Model file for the job. Use its own axes, mm. Face numbers are marked on the shaded views. A direction names the side the tool comes from. Round coordinates to 2 decimals unless told otherwise and drop trailing zeros. Order: outer loops, then holes, each group sorted by start corner. A loop starts at its lowest first (then second) coordinate and runs counter-clockwise, first axis right, second up. Notation, with made-up numbers: M 82,79.5 L 119,79.5 A28 ccw 119,104.5 Z; hole C 38.5,78 d7. An arc over 180 degrees is marked long. Return JSON: item names as keys, results as strings. Group by question number.
Item 1: Slice it at C-C on z = 10. Write the cut outline in (x, y), then the cut area to 3 significant figures.
Item 2: Slice it at D-D on x = 19. Write the cut outline in (y, z).
Item 3: Slice it at B-B on x = 40. Write the cut outline in (y, z), then the cut area to 3 significant figures.
Item 4: Pin check, flat tips, straight feed: pin 1 Ø2 at (x, z) = (10, 5) entering from +Y; pin 2 Ø8 at (x, z) = (0, 0) entering from +Y; pin 3 Ø1.8 at (x, z) = (1, 1) entering from +Y. Stop position of each tip, or through.
Item 5: Which spindle directions (+Z, -Z, +X, -X, +Y, -Y) get a long thin tool onto all of the face, cutting with end or side? Do the marked faces 1, 2, 3 and 4. Say none if no direction does.
Item 6: Slice it at A-A on y = 2.5. Write the cut outline in (x, z), then the cut area to 3 significant figures.
Item 7: Probe line 1 along X through (y, z) = (4.7, 0); line 2 along X through (y, z) = (4.45, 0); line 3 along Z through (x, y) = (40, 1.65). List the from-to ranges inside material, lowest first.
Item 8: Pull direction X, two halves, no side cores. Call the marked faces 5, 6, 7 and 8: pulls with the +X half, pulls with the -X half, needs draft (parallel to the pull), parting line crosses it, or undercut.
from build123d import *

# Parameters (mm, degrees)
EXTRUDE_1_DEPTH     = 4
SKETCH_2_R          = 4.5
SKETCH_2_R_2        = 3
EXTRUDE_2_DEPTH     = 2.5
EXTRUDE_3_DEPTH     = 25
SKETCH_4_W          = 7
SKETCH_4_H          = 5
CUT_EXTRUDE_1_DEPTH = 57.621550668
SKETCH_5_W          = 7
SKETCH_5_H          = 5
CUT_EXTRUDE_2_DEPTH = 52.780787943
EXTRUDE_4_DEPTH     = 2
SKETCH_7_R          = 3
SKETCH_7_R_2        = 1.5
EXTRUDE_5_DEPTH     = 1


with BuildPart() as part:
    # 草图1 → 凸台-拉伸1 (new body)
    with BuildSketch(Plane(origin=(0, 0, 0), x_dir=(1, 0, 0), z_dir=(0, 1, 0))):
        with BuildLine():
            ThreePointArc((12.5, 0), (8.838834765, 8.838834765), (0, 12.5))
            ThreePointArc((0, 12.5), (-8.838834765, 8.838834765), (-12.5, 0))
            Line((-12.5, 0), (-1.5, 0))
            ThreePointArc((-1.5, 0), (0, 1.5), (1.5, 0))
            Line((1.5, 0), (12.5, 0))
        make_face()
        with BuildLine():
            ThreePointArc((0, -12.5), (8.838834765, -8.838834765), (12.5, 0))
            Line((12.5, 0), (1.5, 0))
            ThreePointArc((1.5, 0), (0, -1.5), (-1.5, 0))
            Line((-1.5, 0), (-12.5, 0))
            ThreePointArc((-12.5, 0), (-8.838834765, -8.838834765), (0, -12.5))
        make_face()
        with BuildLine():
            Line((50, 12.5), (0, 12.5))
            ThreePointArc((0, 12.5), (8.838834765, 8.838834765), (12.5, 0))
            Line((12.5, 0), (38.5, 0))
            ThreePointArc((38.5, 0), (40, 1.5), (41.5, 0))
            Line((41.5, 0), (50, 0))
            Line((50, 0), (50, 12.5))
        make_face()
        with BuildLine():
            Line((38.5, 0), (12.5, 0))
            ThreePointArc((12.5, 0), (8.838834765, -8.838834765), (0, -12.5))
            Line((0, -12.5), (50, -12.5))
            Line((50, -12.5), (50, 0))
            Line((50, 0), (41.5, 0))
            ThreePointArc((41.5, 0), (40, -1.5), (38.5, 0))
        make_face()
    extrude(amount=EXTRUDE_1_DEPTH)

    # 草图2 → 凸台-拉伸2 (add)
    with BuildSketch(Plane(origin=(0, 4, 0), x_dir=(1, 0, 0), z_dir=(0, 1, 0))):
        with Locations(Location((0, 0, 0), (0, 0, 270))):
            Circle(SKETCH_2_R)
        with Locations(Location((0, 0, 0), (0, 0, 270))):
            Circle(SKETCH_2_R_2, mode=Mode.SUBTRACT)
    extrude(amount=EXTRUDE_2_DEPTH)

    # 草图3 → 凸台-拉伸3 (add)
    with BuildSketch(Plane.XY.offset(12.5)):
        Polygon((33, 9), (47, 9), (50, 4), (30, 4), align=None)
    extrude(amount=-EXTRUDE_3_DEPTH)

    # 草图4 → 切除-拉伸1 (cut, through all)
    with BuildSketch(Plane.XY.offset(12.5)):
        with Locations((40, 6.5)):
            Rectangle(SKETCH_4_W, SKETCH_4_H)
    extrude(amount=-CUT_EXTRUDE_1_DEPTH, mode=Mode.SUBTRACT)

    # 草图5 → 切除-拉伸2 (cut, through all)
    with BuildSketch(Plane(origin=(0, 4, 0), x_dir=(1, 0, 0), z_dir=(0, 1, 0))):
        with Locations((40, -10)):
            Rectangle(SKETCH_5_W, SKETCH_5_H)
        with Locations((40, 10)):
            Rectangle(SKETCH_5_W, SKETCH_5_H)
    extrude(amount=-CUT_EXTRUDE_2_DEPTH, mode=Mode.SUBTRACT)

    # 草图6 → 凸台-拉伸4 (add, symmetric)
    with BuildSketch(Plane.XY):
        Polygon((30, 4), (33, 9), (4.5, 6.5), (3.215772895, 6.5), (3.215772895, 4), align=None)
    extrude(amount=EXTRUDE_4_DEPTH, both=True)

    # 草图7 → 凸台-拉伸5 (add)
    with BuildSketch(Plane(origin=(0, 4, 0), x_dir=(1, 0, 0), z_dir=(0, 1, 0))):
        with Locations(Location((0, 0, 0), (0, 0, 270))):
            Circle(SKETCH_7_R)
        with Locations(Location((0, 0, 0), (0, 0, 270))):
            Circle(SKETCH_7_R_2, mode=Mode.SUBTRACT)
    extrude(amount=EXTRUDE_5_DEPTH)


solid = part.part
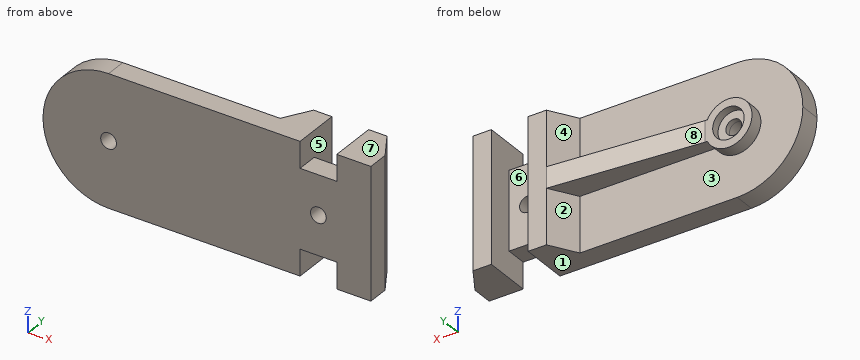
Output values:
{
 "1": {"outline": "M -7.5,0 L 36.5,0 L 36.5,9 L 33,9 L 30,4 L -7.5,4 Z; M 43.5,0 L 50,0 L 50,4 L 47,9 L 43.5,9 Z", "area": "252 mm²"},
 "2": {"outline": "M 0,-12.5 L 4,-12.5 L 4,-2 L 7.77,-2 L 7.77,2 L 4,2 L 4,12.5 L 0,12.5 Z"},
 "3": {"outline": "M 0,-7.5 L 4,-7.5 L 4,-1.5 L 0,-1.5 Z; M 0,1.5 L 4,1.5 L 4,7.5 L 0,7.5 Z", "area": "48.0 mm²"},
 "4": {"pin 1": "y = 4", "pin 2": "y = 6.5", "pin 3": "y = 5"},
 "5": {"face 1": "-Z, +X, -X, +Y, -Y", "face 2": "-Z, +Y", "face 3": "+Y", "face 4": "+Z, +Y"},
 "6": {"outline": "M 0,-12.5 L 36.5,-12.5 L 36.5,-7.5 L 43.5,-7.5 L 43.5,-12.5 L 50,-12.5 L 50,12.5 L 43.5,12.5 L 43.5,7.5 L 36.5,7.5 L 36.5,12.5 L 0,12.5 A12.5 ccw Z; hole C 0,0 d3; hole C 40,0 d3", "area": "1,410 mm²"},
 "7": {"line 1": "-4.5 to -1.5, 1.5 to 36.5, 43.5 to 49.58", "line 2": "-4.5 to -1.5, 1.5 to 36.5, 43.5 to 49.73", "line 3": "-7.5 to -1.5, 1.5 to 7.5"},
 "8": {"face 5": "undercut", "face 6": "undercut", "face 7": "needs draft", "face 8": "pulls with the -X half"}
}
